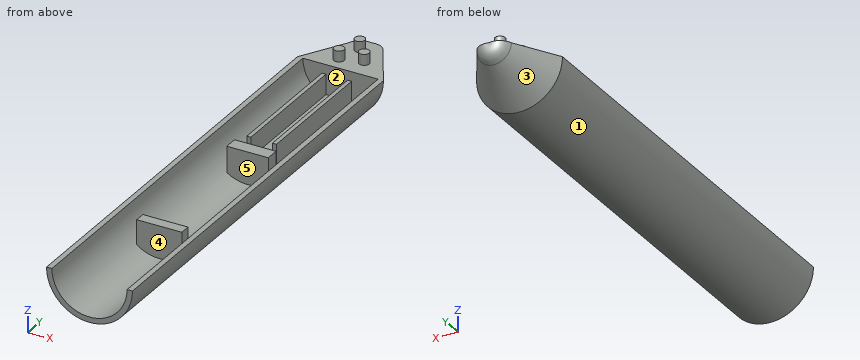
from build123d import *

# Parameters (mm, degrees)
SKETCH2_W                = 2
SKETCH2_H                = 162.039928857
SKETCH5_W                = 72.783621468
SKETCH5_H                = 192.84631039
CUT_EXTRUDE1_DEPTH       = 94.869329042
BOSS_EXTRUDE1_REACH      = 97.869
BOSS_EXTRUDE1_END_RADIUS = 14
BOSS_EXTRUDE1_START      = -2
SKETCH4_W                = 15.457813272
SKETCH4_H                = 5
SKETCH4_W_2              = 16.763190872
SKETCH4_H_2              = 4
SKETCH4_W_3              = 1.5
SKETCH4_H_3              = 48.554461885
BOSS_EXTRUDE2_REACH      = 105.369
BOSS_EXTRUDE2_START      = -9.5
SKETCH4_4_W              = 8
SKETCH4_4_H              = 48.554461885
SKETCH6_R                = 1.9
BOSS_EXTRUDE3_DEPTH      = 4


with BuildPart() as part:
    # Sketch1 → Revolve1 (revolve)
    with BuildSketch(Plane.XY, mode=Mode.PRIVATE) as revolve1_sk:
        with BuildLine():
            Line((6.354000149, 87.279039692), (16, 71))
            Line((16, 71), (0, 71))
            Line((0, 71), (0, 91))
            add(Edge.make_bspline(
                [(0, 91), (4.668589185, 91.723642341), (6.354000149, 87.279039692)],
                knots=[0, 0, 0, 1, 1, 1], degree=2))
        make_face()
    revolve(revolve1_sk.sketch.rotate(Axis((0, 91, 0), (0, -1, 0)), 180), axis=Axis((0, 91, 0), (0, -1, 0)))

    # Sketch2 → Revolve2 (revolve)
    with BuildSketch(Plane.XY, mode=Mode.PRIVATE) as revolve2_sk:
        with Locations((15, -10.019964429)):
            Rectangle(SKETCH2_W, SKETCH2_H)
    revolve(revolve2_sk.sketch.rotate(Axis((0, 91, 0), (0, -1, 0)), 180), axis=Axis((0, 91, 0), (0, -1, 0)))

    # Sketch5 → Cut-Extrude1 (cut, through all)
    with BuildSketch(Plane.XY):
        Rectangle(SKETCH5_W, SKETCH5_H)
    extrude(amount=CUT_EXTRUDE1_DEPTH, mode=Mode.SUBTRACT)

    # Boss-Extrude1: up to this cylinder (the profile starts inside it)
    boss_extrude1_end = Plane(origin=(0, 0.172402, 0), z_dir=(0, 1, 0)) * Cylinder(BOSS_EXTRUDE1_END_RADIUS, 313.082804, mode=Mode.PRIVATE)
    # Sketch4 → Boss-Extrude1 (add, up to the surface)
    with BuildSketch(Plane.XY.offset(BOSS_EXTRUDE1_START), mode=Mode.PRIVATE) as boss_extrude1_sk1:
        with Locations((0, 13.5)):
            Rectangle(SKETCH4_W, SKETCH4_H)
    boss_extrude1_tool1 = extrude(boss_extrude1_sk1.sketch, amount=-BOSS_EXTRUDE1_REACH, mode=Mode.PRIVATE) & boss_extrude1_end
    add(boss_extrude1_tool1.solids().sort_by_distance((0, 13.5, -2))[0])
    # Sketch4 → Boss-Extrude1 (add, up to the surface)
    with BuildSketch(Plane.XY.offset(BOSS_EXTRUDE1_START), mode=Mode.PRIVATE) as boss_extrude1_sk2:
        with Locations((0, -44)):
            Rectangle(SKETCH4_W_2, SKETCH4_H_2)
    boss_extrude1_tool2 = extrude(boss_extrude1_sk2.sketch, amount=-BOSS_EXTRUDE1_REACH, mode=Mode.PRIVATE) & boss_extrude1_end
    add(boss_extrude1_tool2.solids().sort_by_distance((0, -44, -2))[0])
    # Sketch4 → Boss-Extrude1 (add, up to the surface)
    with BuildSketch(Plane.XY.offset(BOSS_EXTRUDE1_START), mode=Mode.PRIVATE) as boss_extrude1_sk3:
        with Locations((4.75, 44.344804049)):
            Rectangle(SKETCH4_W_3, SKETCH4_H_3)
    boss_extrude1_tool3 = extrude(boss_extrude1_sk3.sketch, amount=-BOSS_EXTRUDE1_REACH, mode=Mode.PRIVATE) & boss_extrude1_end
    add(boss_extrude1_tool3.solids().sort_by_distance((4.75, 44.344804, -2))[0])
    # Sketch4 → Boss-Extrude1 (add, up to the surface)
    with BuildSketch(Plane.XY.offset(BOSS_EXTRUDE1_START), mode=Mode.PRIVATE) as boss_extrude1_sk4:
        with Locations((-4.75, 44.344804049)):
            Rectangle(SKETCH4_W_3, SKETCH4_H_3)
    boss_extrude1_tool4 = extrude(boss_extrude1_sk4.sketch, amount=-BOSS_EXTRUDE1_REACH, mode=Mode.PRIVATE) & boss_extrude1_end
    add(boss_extrude1_tool4.solids().sort_by_distance((-4.75, 44.344804, -2))[0])

    # Sketch4<4> → Boss-Extrude2 (add, up to next)
    with BuildSketch(Plane.XY.offset(BOSS_EXTRUDE2_START), mode=Mode.PRIVATE) as boss_extrude2_sk1:
        with Locations((0, 44.344804049)):
            Rectangle(SKETCH4_4_W, SKETCH4_4_H)
    boss_extrude2_tool1 = extrude(boss_extrude2_sk1.sketch, amount=-BOSS_EXTRUDE2_REACH, mode=Mode.PRIVATE) - part.part
    add(boss_extrude2_tool1.solids().sort_by_distance((0, 44.344804, -9.5))[0])

    # Sketch6 → Boss-Extrude3 (add)
    with BuildSketch(Plane.XY):
        with Locations((4.579301858, 78.367512537)):
            Circle(SKETCH6_R)
        with Locations((-3.558513385, 76.255407818)):
            Circle(SKETCH6_R)
        with Locations((-0.919296183, 85.076551058)):
            Circle(SKETCH6_R)
    extrude(amount=BOSS_EXTRUDE3_DEPTH)


solid = part.part
For this review, take the finished solid that the model builds, in its own axes (mm). Face numbers are marked on the shaded views. A direction names the side the tool comes from. Coordinates: 2 decimals unless noted, no trailing zeros. Loops run counter-clockwise (first coordinate to the right, second up) from the corner with the lowest first, then second, coordinate; pieces in that order, holes last. Notation, with made-up numbers: (32, 49.25) - (62, 49.25) arc R4 ccw to (62, 53.25) - close; hole circle Ø1 at (-11, 22.5). An arc over 180 degrees is marked (long way). Use a Markdown table: item, result. Add a question column.
Item 1: For line 1 (X direction, y = 43, z = -10.25); line 2 (Y direction, x = 3, z = -10.75); line 3 (Y direction, x = 0, z = -4), list the stretches that pass through material, from the lowest coordinate up.
Item 2: Mouldability with a two-part tool opening along X and no side actions: class the marked faces 1 and 2 as pulls with the +X half, pulls with the -X half, needs draft (parallel to the pull), parting line crosses it, or undercut.
Item 3: We need section C-C (y = 0). Give the boundary of the cut face in (x, z).
Item 4: We need section B-B (z = -8). Give the number of separate pieces and of enclosed holes in the cut face, and give its area (3 significant figures).
Item 5: Tool access review of the marked faces 3, 4 and 5: name each direction out of +Z, -Z, +X, -X, +Y, -Y from which nothing blocks a thin tool from reaching the whole face with its end or side.
Item 6: Insertion check: pin 1 Ø1.5 at (y, z) = (14, -4.5) entering from -X; pin 2 Ø0.8 at (x, y) = (-4.5, 49) entering from +Z; pin 3 Ø4 at (x, y) = (0.5, -65.5) entering from -Z; pin 4 Ø1 at (x, z) = (-6, -13) entering from +Y. Each pin has a flat end and moves straight along its axis. Give the tip position at first contact, or say it passes through.
Item 7: We need section A-A (y = 27). Give the boundary of the cut face in (x, z), and give its area (3 significant figures).
Results list:
| question | item | result |
|---|---|---|
| 1 | line 1 | x = -12.29 to -9.54, -5.5 to 5.5, 9.54 to 12.29 |
| 1 | line 2 | y = -46 to -42, 11 to 16, 20.07 to 68.62, 71 to 79.17 |
| 1 | line 3 | y = -46 to -42, 11 to 16, 71 to 90.39 |
| 2 | face 1 | parting line crosses it |
| 2 | face 2 | undercut |
| 3 | outline | (-16, 0) arc R16 ccw to (16, 0) - (14, 0) arc R14 cw to (-14, 0) - close |
| 4 | separate pieces | 5 |
| 4 | enclosed holes | 0 |
| 4 | area | 1,290 mm^2 |
| 5 | face 3 | -Z, +Y |
| 5 | face 4 | +Z, -Y |
| 5 | face 5 | +Z |
| 6 | pin 1 | stops at x = -15.55 |
| 6 | pin 2 | stops at z = -2 |
| 6 | pin 3 | stops at z = -16 |
| 6 | pin 4 | stops at y = 74.68 |
| 7 | outline | (-16, 0) arc R16 ccw to (16, 0) - (14, 0) arc R14 cw to (5.5, -12.87) - (5.5, -2) - (4, -2) - (4, -9.5) - (-4, -9.5) - (-4, -2) - (-5.5, -2) - (-5.5, -12.87) arc R14 cw to (-14, 0) - close |
| 7 | area | 162 mm^2 |
